Here's how the part is built. I have some questions about the finished solid (model axes, mm). A direction names the side the tool comes from. Coordinates: 2 decimals unless noted, no trailing zeros. Write each loop counter-clockwise with the first axis right and the second up, starting at its lowest first coordinate (ties: lowest second). Pieces come first, ordered by that corner, then holes. Notation, with made-up numbers: (-35.75, 39) - (22.25, 39) arc R20 cw to (22.25, 60) - close; hole circle Ø7 at (20.25, 1.25). An arc over 180 degrees is marked (long way). Answer in a Markdown table with one row per item. Add a question column.
Item 1: Imagine slicing it at D-D (x = 0). Please give me the cut outline in (y, z) (1 decimal), plus the area to 3 significant figures.
Item 2: Imagine slicing it at C-C (z = 0). Please give me the cut outline in (x, y).
Item 3: Which directions (+Z, -Z, +X, -X, +Y, -Y) give clear straight access to the entire face, cutting with the end or side of a thin tool? Please do faces 1 (the face through (5.752, 2.557, 12.298)), 2 (the face through (-3.435, 0.022, 15.146)), 3 (the face through (8.137, 2.016, 22.887)), 4 (the face through (0.04, 1.94, 2.54)).
Item 4: If I drill on probe 1 along X at (y, z) = (0.95, 25.4); probe 2 along Z at (x, y) = (0, -0.6) (3 decimals); probe 3 along Z at (x, y) = (1, -0.45) (3 decimals), over which ranges is the centre line in solid material (lowest first)? Write a range as from..to.
Item 5: Imagine slicing it at B-B (z = 25.4). Please give me the cut outline in (x, y).
Item 6: I'm going to push flat-ended pins straight in: pin 1 (2.5 mm diameter, centred on x = -1, y = 0.5, fed in from -Z) (3 decimals); pin 2 (2 mm diameter, centred on y = -0.5, z = 4.5, fed in from -X); pin 3 (1.6 mm diameter, centred on x = 7.77, z = 25.4, fed in from -Y); pin 4 (6 mm diameter, centred on x = -2.5, z = 24.5, fed in from +Y). Where does each tip first touch, or does it pass through?
Item 7: We'd pull the mould along X, two halves only. Please class faces 5 (the face through (-7.94, -0.02, 24.04)), 6 (the face through (0.057, 0.022, -3.174)), 7 (the face through (-5, -1.588, 16)): +X half, -X half, draft (parallel to the pull), parting line (faces both ways), or undercut.
Item 8: Imagine slicing it at A-A (y = 1.2). State how many separate pieces and enclosed holes the cut face has, plus the area to 3 significant figures.
from build123d import *

# Parameters (mm, degrees)
SKETCH1_R        = 1.3716
BODY_DEPTH       = 1.5875
SKETCH2_R        = 1.3716
RIB_DEPTH        = 3.175
ANGLE_DEPTH      = 11.940559309
ANGLE_DEPTH_BACK = 11.940559309
BOLT_START       = -3.175
SKETCH5_R        = 2.54
BOLT_HOLE_DEPTH  = 2.54


with BuildPart() as part:
    # Sketch1 → Body (new body, symmetric)
    with BuildSketch(Plane(origin=(0, 0, 0), x_dir=(1, 0, 0), z_dir=(0, 1, 0))):
        with BuildLine():
            Line((-3.0362676, 0.928280162), (-10.801826909, -24.471719838))
            ThreePointArc((-10.801826909, -24.471719838), (-10.317804842, -27.288562348), (-7.765559309, -28.575))
            Line((-7.765559309, -28.575), (7.765559309, -28.575))
            ThreePointArc((7.765559309, -28.575), (10.317804842, -27.288562348), (10.801826909, -24.471719838))
            Line((10.801826909, -24.471719838), (3.0362676, 0.928280162))
            ThreePointArc((3.0362676, 0.928280162), (0, 3.175), (-3.0362676, 0.928280162))
        make_face()
        Circle(SKETCH1_R, mode=Mode.SUBTRACT)
        with Locations((-7.765559309, -25.4)):
            Circle(SKETCH1_R, mode=Mode.SUBTRACT)
        with Locations((7.765559309, -25.4)):
            Circle(SKETCH1_R, mode=Mode.SUBTRACT)
        with BuildLine():
            Line((-1.21450704, -7.88188057), (-5.719084006, -22.615687935))
            ThreePointArc((-5.719084006, -22.615687935), (-5.525475179, -23.742424939), (-4.504576966, -24.257))
            Line((-4.504576966, -24.257), (4.504576966, -24.257))
            ThreePointArc((4.504576966, -24.257), (5.525475179, -23.742424939), (5.719084006, -22.615687935))
            Line((5.719084006, -22.615687935), (1.21450704, -7.88188057))
            ThreePointArc((1.21450704, -7.88188057), (0, -6.983192635), (-1.21450704, -7.88188057))
        make_face(mode=Mode.SUBTRACT)
    extrude(amount=BODY_DEPTH, both=True)

    # Sketch2 → Rib (add)
    with BuildSketch(Plane(origin=(0, 1.5875, 0), x_dir=(1, 0, 0), z_dir=(0, 1, 0))):
        with BuildLine():
            Line((-7.487715721, -24.056836011), (-6.933591046, -22.24437587))
            Line((-6.933591046, -22.24437587), (-2.42901408, -7.510568505))
            ThreePointArc((-2.42901408, -7.510568505), (0, -5.713192635), (2.42901408, -7.510568505))
            Line((2.42901408, -7.510568505), (6.933591046, -22.24437587))
            Line((6.933591046, -22.24437587), (7.487715721, -24.056836011))
            ThreePointArc((7.487715721, -24.056836011), (8.631641376, -24.336426583), (9.137159309, -25.4))
            ThreePointArc((9.137159309, -25.4), (8.904756482, -26.163882426), (8.286304306, -26.668901576))
            Line((8.286304306, -26.668901576), (8.442739025, -27.180576489))
            ThreePointArc((8.442739025, -27.180576489), (9.476466758, -26.237747397), (9.587319869, -24.843031903))
            Line((9.587319869, -24.843031903), (1.82176056, 0.556968097))
            ThreePointArc((1.82176056, 0.556968097), (0, 1.905), (-1.82176056, 0.556968097))
            Line((-1.82176056, 0.556968097), (-9.587319869, -24.843031903))
            ThreePointArc((-9.587319869, -24.843031903), (-9.476466758, -26.237747397), (-8.442739025, -27.180576489))
            Line((-8.442739025, -27.180576489), (-8.286304306, -26.668901576))
            ThreePointArc((-8.286304306, -26.668901576), (-9.077226912, -24.99898297), (-7.487715721, -24.056836011))
        make_face()
        Circle(SKETCH2_R, mode=Mode.SUBTRACT)
    extrude(amount=RIB_DEPTH)

    # Sketch6 → Angle (cut, two sides)
    with BuildSketch(Plane(origin=(0, 0, 0), x_dir=(0, 0, -1), z_dir=(1, 0, 0))) as angle_sk:
        Polygon((-14.480576489, 4.1275), (2.051640081, 1.5875), (2.051640081, 8.789734229), (-27.180576489, 8.789734229), (-27.180576489, 1.5875), align=None)
    extrude(amount=ANGLE_DEPTH, mode=Mode.SUBTRACT)
    extrude(angle_sk.sketch, amount=-ANGLE_DEPTH_BACK, mode=Mode.SUBTRACT)

    # Sketch5 → Bolt hole (cut)
    with BuildSketch(Plane.XZ.offset(1.5875).offset(BOLT_START)):
        Circle(SKETCH5_R)
        with Locations((7.765559309, 25.4)):
            Circle(SKETCH5_R)
        with Locations((-7.765559309, 25.4)):
            Circle(SKETCH5_R)
    extrude(amount=-BOLT_HOLE_DEPTH, mode=Mode.SUBTRACT)


solid = part.part
Here are the results:
| question | item | result |
|---|---|---|
| 1 | outline | (-1.6, -3.2) - (1.6, -3.2) - (1.6, -1.4) - (-1.6, -1.4) - close; (-1.6, 1.4) - (1.6, 1.4) - (1.6, 2.5) - (2.3, 2.5) - (2.8, 5.7) - (1.6, 5.7) - (1.6, 7) - (-1.6, 7) - close; (-1.6, 24.3) - (1.6, 24.3) - (1.6, 28.6) - (-1.6, 28.6) - close |
| 1 | area | 40.3 mm2 |
| 2 | outline | (-3.32, -1.59) - (-1.37, -1.59) - (-1.37, 1.59) - (-3.32, 1.59) - close; (1.37, -1.59) - (3.32, -1.59) - (3.32, 1.59) - (1.37, 1.59) - close |
| 3 | face 1 | -Z, +X, +Y |
| 3 | face 2 | +Y, -Y |
| 3 | face 3 | +Z, +Y |
| 3 | face 4 | -Z, +Y |
| 4 | probe 1 | x = -10.94..-9.14, -6.39..6.39, 9.14..10.94 |
| 4 | probe 2 | z = -3.175..-1.372, 1.372..6.983, 24.257..28.575 |
| 4 | probe 3 | z = -3.013..-0.939, 0.939..7.47, 24.257..28.575 |
| 5 | outline | (-10.94, -1.59) - (-9.14, -1.59) - (-9.14, 1.59) - (-10.94, 1.59) - close; (-6.39, -1.59) - (6.39, -1.59) - (6.39, 1.59) - (-6.39, 1.59) - close; (9.14, -1.59) - (10.94, -1.59) - (10.94, 1.59) - (9.14, 1.59) - close |
| 6 | pin 1 | stops at z = -3.175 |
| 6 | pin 2 | stops at x = -5 |
| 6 | pin 3 | passes through |
| 6 | pin 4 | stops at y = 1.59 |
| 7 | face 5 | undercut |
| 7 | face 6 | parting line |
| 7 | face 7 | draft |
| 8 | separate pieces | 1 |
| 8 | enclosed holes | 4 |
| 8 | area | 307 mm2 |
